Autodesk Inventor part; units mm, degrees
ref_plane "YZ Plane" through (0, 0, 0) normal (1, 0, 0) x (0, 1, 0)
ref_plane "XZ Plane" through (0, 0, 0) normal (0, 1, 0) x (-1, 0, 0)
ref_plane "XY Plane" through (0, 0, 0) normal (0, 0, 1) x (1, 0, 0)
sketch "Szkic1" plane through (0, 0, 0) normal (0, 1, 0) x (-1, 0, 0)
  line L0 (0, 0) -> (-12, 0)
  line L1 (-12, 0) -> (-12, -26)
  line L2 (-12, -26) -> (0, -26)
  line L3 (0, -26) -> (0, 0)
  line L4 (-12, 0) -> (-42, -4)
  line L5 (-42, -4) -> (-42, -22)
  line L6 (-42, -22) -> (-12, -26)
  circle A0 centre (-34, -13) radius 5
  line L7 (-34, -18) -> (-42, -18)
  line L8 (-34, -8) -> (-42, -8)
  dimension "d0" = 12
  dimension "d1" = 26
  dimension "d2" = 18
  dimension "d3" = 30
  dimension "d4" = 10
extrude "Wyciągnięcie proste1" add sketch "Szkic1" along normal blind 7 contours L3 L2 L1 L0 | L1 L6 L5 L7 A0 L8 L4
sketch "Szkic2" plane through (0, 7, 0) normal (0, 1, 0) x (1, 0, 0)
  line L0 (0, 26) -> (0, 0)
  line L1 (0, 26) -> (7, 26)
  line L2 (7, 26) -> (7, 0)
  line L3 (7, 0) -> (0, 0)
  line L4 (0, 0) -> (0, 26)
extrude "Wyciągnięcie proste2" add sketch "Szkic2" along normal blind 21
sketch "Szkic3" plane through (0, 0, -26) normal (-1, 0, 0) x (0, 0, 1)
  line L0 (8, 28) -> (18, 28)
  line L1 (18, 28) -> (18, 0)
  line L2 (18, 0) -> (8, 0)
  line L3 (8, 0) -> (8, 28)
  line L4 (0, 0) -> (0, 28)
  point P0 (26, 0)
  dimension "d9" = 10
  dimension "d10" = 8
extrude "Wyciągnięcie proste3" add sketch "Szkic3" along normal blind 28
sketch "Szkic4" plane through (0, 0, -8) normal (0, 0, 1) x (1, 0, 0)
  point P0 (0, 0)
  point P1 (-14, 14)
hole "Otwór1" at (-14, 14, -8) direction (0, 0, -1) diameter 14 end through all
full round fillet "Zaokrąglenie pełne1" first side at (-18.6667, 28, -14.6667) centre faces at (-28, 18.6667, -14.6667) second side at (17.6788, 0, -13.2009)
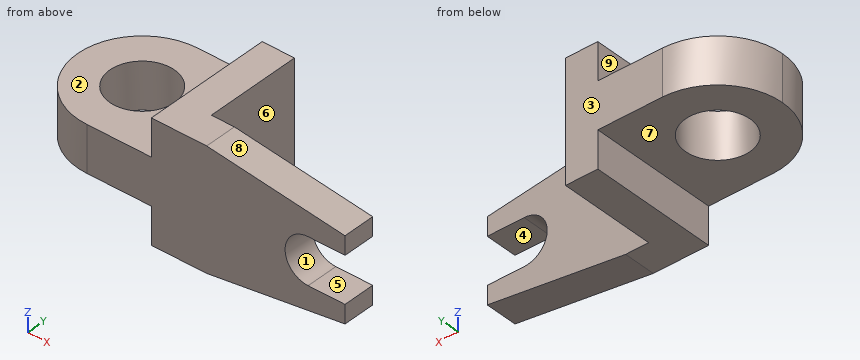
The listing builds one solid part. Answer for the finished solid, in the listing's coordinates (mm). Face numbers are marked on the shaded views. A direction names the side the tool comes from. Give positions to 0.01 mm unless a question says otherwise; leave off trailing zeros. Loops run counter-clockwise (first coordinate to the right, second up) from the corner with the lowest first, then second, coordinate; pieces in that order, holes last. Notation, with made-up numbers: M 38,60 L 46,60 A14 ccw 46,73 Z; hole C 87,89 d9. An arc over 180 degrees is marked long. One line per item, written item: value.
Q1. Find the intervals of material crossed by line 1 (Y direction, x = -14, z = -15.75); line 2 (X direction, y = 14, z = -13.5); line 3 (Z direction, x = -20, y = 19.5), in increasing order. Write a range as from..to.
Working result:
line 1: y = 0..7, 21..28
line 2: x = -28..-21, -7..7
line 3: z = -18..-8
Q2. A cutting plane is placed at A-A on y = 9.75. Determine the outline of the cut face in (x, z).
Working result:
outline: M -27.34,-18 L -19.56,-18 L -19.56,-8 L -27.34,-8 Z; M -8.44,-18 L 0,-18 L 0,-26 L 7,-26 L 7,0 L 0,0 L 0,-8 L -8.44,-8 Z
Q3. Flat-ended cylindrical pins translate along their axes: P1, Ø5, axis at x = 22.5, z = -5.5, coming from the -Y side; P2, Ø9, axis at y = 9.5, z = -23.5, coming from the -X side; P3, Ø3.5, axis at x = 38, y = 2, coming from the +Z side; P4, Ø5.5, axis at x = 39.5, y = 5, coming from the -Z side. Find the tip coordinate at first contact, or state that the pin passes through.
Working result:
P1: stops at y = 0
P2: stops at x = 0
P3: stops at z = -3.23
P4: stops at z = -22.7
Q4. Determine the mould class of the marked faces 1, 2, 3 and 4 for opening direction Z: +Z half, -Z half, draft (parallel to the pull), parting line (faces both ways), or undercut.
Working result:
face 1: undercut
face 2: +Z half
face 3: draft
face 4: undercut
Q5. A cutting plane is placed at C-C on z = -23.5. Determine the outline of the cut face in (x, y).
Working result:
outline: M 0,0 L 30.75,0 L 30.75,7 L 7,7 L 7,28 L 0,28 Z
Q6. A cutting plane is placed at D-D on y = 26.25. Determine the outline of the cut face in (x, z).
Working result:
outline: M -20.78,-18 L 0,-18 L 0,-26 L 7,-26 L 7,0 L 0,0 L 0,-8 L -20.78,-8 Z
Q7. For the marked faces 5, 6, 7, 8 and 9, determine the directions among +Z, -Z, +X, -X, +Y, -Y from which every point of the face is accessible in a straight line to the end or side of a thin tool.
Working result:
face 5: +X, +Y, -Y
face 6: +Z, -Z, +X, +Y
face 7: -Z, -X, +Y, -Y
face 8: +Z, +X, +Y, -Y
face 9: +Z, -X, +Y, -Y
